Model file for the job. Use its own axes, mm. Face numbers are marked on the shaded views. A direction names the side the tool comes from. Give positions to 0.01 mm unless a question says otherwise; leave off trailing zeros. Order: outer loops, then holes, each group sorted by start corner. A loop starts at its lowest first (then second) coordinate and runs counter-clockwise, first axis right, second up. Notation, with made-up numbers: (5, 60.5) - (12, 60.5) arc R17 ccw to (12, 73.5) - close; hole circle Ø4 at (15.5, 59.25). An arc over 180 degrees is marked (long way). Return JSON: item names as keys, results as strings. Group by question number.
from build123d import *

# Parameters (mm, degrees)
F1_DEPTH        = 16
F2_R            = 11
F3_DEPTH        = 26
F4_R            = 8.75
F5_DEPTH        = 40
F7_D            = 9
F7_DEPTH        = 35
F7_TIP          = 2.7038727856
F8_R            = 2.7
F9_DEPTH        = 12.5
F11_D           = 3
F11_CBORE_D     = 6
F11_CBORE_DEPTH = 5


with BuildPart() as f1:
    # F0 (on Top) → F1 (new body)
    with BuildSketch(Plane.XY):
        with BuildLine():
            ThreePointArc((0.78, -12.976578902), (9.4641428561, -8.9123509805), (13, 0))
            ThreePointArc((13, 0), (9.4641428561, 8.9123509805), (0.78, 12.976578902))
            ThreePointArc((0.78, 12.976578902), (-13, 0), (0.78, -12.976578902))
        make_face()
        with BuildLine():
            ThreePointArc((0.78, 12.976578902), (9.4641428561, 8.9123509805), (13, 0))
            ThreePointArc((13, 0), (9.4641428561, -8.9123509805), (0.78, -12.976578902))
            Line((0.78, -12.976578902), (50.6, -9.9819837708))
            ThreePointArc((50.6, -9.9819837708), (40, 0), (50.6, 9.9819837708))
            Line((50.6, 9.9819837708), (0.78, 12.976578902))
        make_face()
        with BuildLine():
            ThreePointArc((60, 0), (57.2801098893, 6.8556546004), (50.6, 9.9819837708))
            ThreePointArc((50.6, 9.9819837708), (40, 0), (50.6, -9.9819837708))
            ThreePointArc((50.6, -9.9819837708), (57.2801098893, -6.8556546004), (60, 0))
        make_face()
    extrude(amount=F1_DEPTH)

    # F2 (on Top) → F3 (join)
    with BuildSketch(Plane.XY):
        Circle(F2_R)
    extrude(amount=F3_DEPTH)

    # F4 (on Top) → F5 (join)
    with BuildSketch(Plane.XY):
        Circle(F4_R)
    extrude(amount=F5_DEPTH)

    # F7
    with Locations(Plane.XY.offset(40)):
        with Locations((0, 0)):
            Hole(F7_D / 2, depth=F7_DEPTH)
            with Locations((0, 0, -(F7_DEPTH + F7_TIP / 2))):  # 118° drill point
                Cone(0, F7_D / 2, F7_TIP, mode=Mode.SUBTRACT)

    # F8 (on Front) → F9 (cut, symmetric)
    with BuildSketch(Plane.XZ):
        with Locations((0, 21)):
            Circle(F8_R)
    extrude(amount=F9_DEPTH, both=True, mode=Mode.SUBTRACT)

    # F11 (through all)
    with Locations(Plane.XY.offset(16)):
        with Locations((50, 0)):
            CounterBoreHole(F11_D / 2, F11_CBORE_D / 2, F11_CBORE_DEPTH)


solid = f1.part
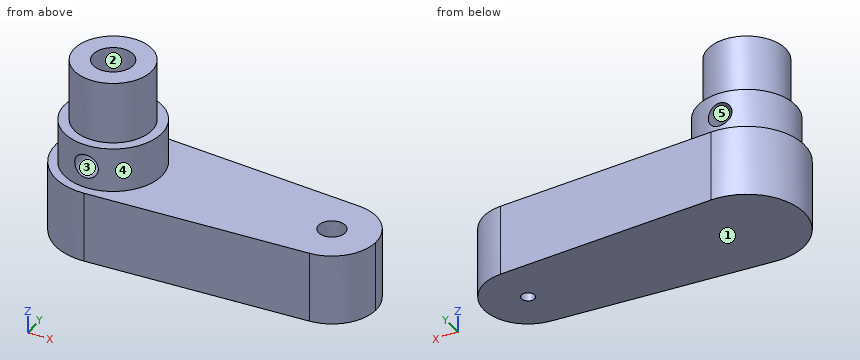
(1) Drop flat-ended pins along their axis: pin 1 Ø4 at (x, y) = (49.5, -3) entering from +Z; pin 2 Ø1.5 at (y, z) = (6.5, 27.5) entering from -X; pin 3 Ø3 at (y, z) = (9, 25.5) entering from +X; pin 4 Ø2.5 at (x, y) = (50, 0) entering from -Z. Give the stop position or say it passes through.
(2) Drill centre lines: L1, parallel to X at y = 0.5, z = 10.5; L2, parallel to Z at x = 0, y = -7; L3, parallel to Z at x = 32, y = 9.5. Where is each one in solid material? Low to high.
(3) Slice it at A-A (z = 6). Give the cut face in (x, y).
(4) 3-axis set-ups, long thin cutter, end or side, ignore diameter. For the marked faces 4 and 5: which of +Z, -Z, +X, -X, +Y, -Y reach the whole face in a straight line?
(5) Slice it at B-B (z = 21). Give the cut face in (x, y), and give its area (3 significant figures).
(6) Slice it at D-D (x = 28). Give the cut face in (y, z), and give its area (3 significant figures).
(7) Slice it at C-C (z = 31.5). Give the cut face in (x, y).
(8) Pull direction Z, two halves, no side cores. Call the marked faces 1, 2 and 3: released by +Z, released by -Z, zero draft, split by the parting line, or undercut.
Result set:
{
 "1": {"pin 1": "stops at z = 16", "pin 2": "stops at x = -6.6", "pin 3": "stops at x = 8.05", "pin 4": "passes through"},
 "2": {"L1": "x = -12.99 to -4.47, 4.47 to 48.59, 51.41 to 59.99", "L2": "z = 0 to 18.3, 23.7 to 40", "L3": "z = 0 to 16"},
 "3": {"outline": "(0.78, -12.98) - (50.6, -9.98) arc R10 ccw to (50.6, 9.98) - (0.78, 12.98) arc R13 ccw (long way) to start; hole circle Ø9 at (0, 0); hole circle Ø3 at (50, 0)"},
 "4": {"face 4": "+Z", "face 5": "+Y, -Y"},
 "5": {"outline": "(-2.7, -10.66) - (-2.7, -3.6) arc R4.5 cw to (-2.7, 3.6) - (-2.7, 10.66) arc R11 ccw to start; (2.7, -10.66) arc R11 ccw to (2.7, 10.66) - (2.7, 3.6) arc R4.5 cw to (2.7, -3.6) - close", "area": "244 mm²"},
 "6": {"outline": "(-11.34, 0) - (11.34, 0) - (11.34, 16) - (-11.34, 16) - close", "area": "363 mm²"},
 "7": {"outline": "circle Ø17.5 at (0, 0); hole circle Ø9 at (0, 0)"},
 "8": {"face 1": "released by -Z", "face 2": "zero draft", "face 3": "undercut"}
}
